from build123d import *

# Parameters (mm, degrees)
SKETCH_1_W                  = 220
SKETCH_1_H                  = 224.25
SKETCH_1_W_2                = 210
SKETCH_1_H_2                = 214.25
EXTRUDE_1_DEPTH             = 310
SKETCH_2_W                  = 280
SKETCH_2_H                  = 284.25
SKETCH_2_W_2                = 210
SKETCH_2_H_2                = 214.25
EXTRUDE_2_DEPTH             = 10
FILLET_1_R                  = 5
FILLET_2_R                  = 5
FILLET_3_R                  = 10
HOLE_WIZARD_8_4_8_4_1_D     = 8.4
MM_11_D                     = 10
HOLE_WIZARD_4_5_4_5_1_D     = 4.5
HOLE_WIZARD_4_5_4_5_1_DEPTH = 5
HOLE_WIZARD_6_6_6_6_1_D     = 6.6
HOLE_WIZARD_6_6_6_6_1_DEPTH = 5
HOLE_WIZARD_5_5_5_5_1_D     = 5.5
HOLE_WIZARD_5_5_5_5_1_DEPTH = 5
CUT_EXTRUDE_1_REACH         = 252
SKETCH_45_W                 = 250
SKETCH_45_H                 = 154.25
FILLET_4_R                  = 5
SKETCH_49_W                 = 256
SKETCH_49_H                 = 160.25
EXTRUDE_3_DEPTH             = 3
FILLET_5_R                  = 5
SKETCH_50_W                 = 216
SKETCH_50_H                 = 220.25
EXTRUDE_4_DEPTH             = 3
FILLET_6_R                  = 5
HOLE_WIZARD_6_4_6_4_1_D     = 6.4
HOLE_WIZARD_6_4_6_4_1_DEPTH = 5
HOLE_WIZARD_4_2_4_2_1_D     = 4.2
HOLE_WIZARD_4_2_4_2_1_DEPTH = 5


with BuildPart() as part:
    # 草图1 → 凸台-拉伸1 (new body)
    with BuildSketch(Plane.XY):
        Rectangle(SKETCH_1_W, SKETCH_1_H)
        Rectangle(SKETCH_1_W_2, SKETCH_1_H_2, mode=Mode.SUBTRACT)
    extrude(amount=EXTRUDE_1_DEPTH)

    # 草图2 → 凸台-拉伸2 (add)
    with BuildSketch(Plane(origin=(0, 0, 0), x_dir=(-1, 0, 0), z_dir=(0, 0, -1))):
        Rectangle(SKETCH_2_W, SKETCH_2_H)
        Rectangle(SKETCH_2_W_2, SKETCH_2_H_2, mode=Mode.SUBTRACT)
    extrude(amount=EXTRUDE_2_DEPTH)

    # 圆角1
    fillet_1_edges = [part.edges().sort_by_distance(p)[0] for p in [
        (110, -112.125, 155),
        (-110, -112.125, 155),
        (-110, 112.125, 155),
        (110, 112.125, 155),
    ]]
    fillet(fillet_1_edges, radius=FILLET_1_R)

    # 圆角2
    fillet_2_edges = [part.edges().sort_by_distance(p)[0] for p in [
        (105, -107.125, 150),
        (105, 107.125, 150),
        (-105, 107.125, 150),
        (-105, -107.125, 150),
    ]]
    fillet(fillet_2_edges, radius=FILLET_2_R)

    # 圆角3
    fillet_3_edges = [part.edges().sort_by_distance(p)[0] for p in [
        (-140, -142.125, -5),
        (-140, 142.125, -5),
        (140, 142.125, -5),
        (140, -142.125, -5),
    ]]
    fillet(fillet_3_edges, radius=FILLET_3_R)

    # Ø8.4 (8.4) 直径孔1 (through all)
    with Locations(Plane.XY):
        with Locations((120, 122.125), (120, -122.125), (-120, -122.125), (-120, 122.125)):
            Hole(HOLE_WIZARD_8_4_8_4_1_D / 2)

    # 大小mm 暗销孔11 (through all)
    with Locations(Plane(origin=(0, 112.125, 0), x_dir=(1, 0, 0), z_dir=(0, 1, 0))):
        with Locations((-75, -165), (-50, -165), (-50, -190), (-75, -190), (50, -190), (50, -165), (75, -165), (75, -190)):
            Hole(MM_11_D / 2)

    # Ø4.5 (4.5) 直径孔1
    with Locations(Plane(origin=(0, 112.125, 0), x_dir=(1, 0, 0), z_dir=(0, 1, 0))):
        with Locations((0, -105), (0, -165), (0, -225), (0, -285)):
            Hole(HOLE_WIZARD_4_5_4_5_1_D / 2, depth=HOLE_WIZARD_4_5_4_5_1_DEPTH)

    # Ø6.6 (6.6) 直径孔1
    with Locations(Plane(origin=(0, -112.125, 0), x_dir=(-1, 0, 0), z_dir=(0, -1, 0))):
        with Locations((19, -105.5), (-19, -105.5)):
            Hole(HOLE_WIZARD_6_6_6_6_1_D / 2, depth=HOLE_WIZARD_6_6_6_6_1_DEPTH)

    # Ø5.5 (5.5) 直径孔1
    with Locations(Plane(origin=(0, -112.125, 0), x_dir=(-1, 0, 0), z_dir=(0, -1, 0))):
        with Locations((15, -280), (-15, -280)):
            Hole(HOLE_WIZARD_5_5_5_5_1_D / 2, depth=HOLE_WIZARD_5_5_5_5_1_DEPTH)

    # 草图45 → 切除-拉伸1 (cut, up to next)
    with BuildSketch(Plane.ZY.offset(110), mode=Mode.PRIVATE) as cut_extrude_1_sk1:
        with Locations((155, 0)):
            Rectangle(SKETCH_45_W, SKETCH_45_H)
    cut_extrude_1_tool1 = extrude(cut_extrude_1_sk1.sketch, amount=-CUT_EXTRUDE_1_REACH, mode=Mode.PRIVATE) & part.part
    add(cut_extrude_1_tool1.solids().sort_by_distance((-110, 0, 155))[0], mode=Mode.SUBTRACT)

    # 圆角4
    fillet_4_edges = [part.edges().sort_by_distance(p)[0] for p in [
        (-107.5, -77.125, 280),
        (-107.5, 77.125, 280),
        (-107.5, 77.125, 30),
        (-107.5, -77.125, 30),
    ]]
    fillet(fillet_4_edges, radius=FILLET_4_R)

    # 草图49 → 凸台-拉伸3 (add)
    with BuildSketch(Plane.ZY.offset(110)):
        with Locations((155, 0)):
            Rectangle(SKETCH_49_W, SKETCH_49_H)
        with BuildLine():
            Line((280, -72.125), (280, 72.125))
            ThreePointArc((280, 72.125), (278.535533906, 75.660533906), (275, 77.125))
            Line((275, 77.125), (35, 77.125))
            ThreePointArc((35, 77.125), (31.464466094, 75.660533906), (30, 72.125))
            Line((30, 72.125), (30, -72.125))
            ThreePointArc((30, -72.125), (31.464466094, -75.660533906), (35, -77.125))
            Line((35, -77.125), (275, -77.125))
            ThreePointArc((275, -77.125), (278.535533906, -75.660533906), (280, -72.125))
        make_face(mode=Mode.SUBTRACT)
    extrude(amount=EXTRUDE_3_DEPTH)

    # 圆角5
    fillet_5_edges = [part.edges().sort_by_distance(p)[0] for p in [
        (-111.5, 80.125, 27),
        (-111.5, -80.125, 27),
        (-111.5, -80.125, 283),
        (-111.5, 80.125, 283),
    ]]
    fillet(fillet_5_edges, radius=FILLET_5_R)

    # 草图50 → 凸台-拉伸4 (add)
    with BuildSketch(Plane(origin=(0, 0, -10), x_dir=(-1, 0, 0), z_dir=(0, 0, -1))):
        Rectangle(SKETCH_50_W, SKETCH_50_H)
        with BuildLine():
            Line((-100, -107.125), (100, -107.125))
            ThreePointArc((100, -107.125), (103.535533906, -105.660533906), (105, -102.125))
            Line((105, -102.125), (105, 102.125))
            ThreePointArc((105, 102.125), (103.535533906, 105.660533906), (100, 107.125))
            Line((100, 107.125), (-100, 107.125))
            ThreePointArc((-100, 107.125), (-103.535533906, 105.660533906), (-105, 102.125))
            Line((-105, 102.125), (-105, -102.125))
            ThreePointArc((-105, -102.125), (-103.535533906, -105.660533906), (-100, -107.125))
        make_face(mode=Mode.SUBTRACT)
    extrude(amount=EXTRUDE_4_DEPTH)

    # 圆角6
    fillet_6_edges = [part.edges().sort_by_distance(p)[0] for p in [
        (108, 110.125, -11.5),
        (108, -110.125, -11.5),
        (-108, -110.125, -11.5),
        (-108, 110.125, -11.5),
    ]]
    fillet(fillet_6_edges, radius=FILLET_6_R)

    # Ø6.4 (6.4) 直径孔1
    with Locations(Plane.ZY.offset(110)):
        with Locations((20, 87.125), (20, -87.125), (290, -87.125), (290, 87.125)):
            Hole(HOLE_WIZARD_6_4_6_4_1_D / 2, depth=HOLE_WIZARD_6_4_6_4_1_DEPTH)

    # Ø4.2 (4.2) 直径孔1
    with Locations(Plane(origin=(0, -107.125, 0), x_dir=(1, 0, 0), z_dir=(0, 1, 0))):
        with Locations((-15, -11.55), (15, -11.55), (15, -41.55), (-15, -41.55)):
            Hole(HOLE_WIZARD_4_2_4_2_1_D / 2, depth=HOLE_WIZARD_4_2_4_2_1_DEPTH)


solid = part.part
Can you work these out from the model? Positions are in its coordinate system, mm. A direction names the side the tool comes from. Coordinates: 2 decimals unless noted, no trailing zeros. Order: outer loops, then holes, each group sorted by start corner. A loop starts at its lowest first (then second) coordinate and runs counter-clockwise, first axis right, second up. Notation, with made-up numbers: (35, -26) -> (82, -26) arc R26 ccw to (82, -8) -> close; hole circle Ø8 at (9, 58.5). An arc over 180 degrees is marked (long way). Use one line per item in the form item = value.
Q1. Imagine slicing it at A-A, the plane x = -50. Give the number of separate pieces and of enclosed holes in the cut face, then the cut area to 3 significant figures.
From the geometry:
separate_pieces = 6
enclosed_holes = 0
area = 3,620 mm²
Q2. We'd pull the mould along Z, two halves only. Please class faces 4 (the face through (55, 110, 165)), 5 (the face through (2, -142.125, -5)): released by +Z, released by -Z, zero draft, split by the parting line, or undercut.
From the geometry:
face_4 = undercut
face_5 = zero draft
Q3. Imagine slicing it at C-C, the plane x = -120. List the corners of the cut face in (y, z) for me (3 decimals).
From the geometry:
outline = (-142.125, -10) -> (-126.325, -10) -> (-126.325, 0) -> (-142.125, 0) -> close; (-117.925, -10) -> (117.925, -10) -> (117.925, 0) -> (-117.925, 0) -> close; (126.325, -10) -> (142.125, -10) -> (142.125, 0) -> (126.325, 0) -> close
Q4. Imagine slicing it at D-D, the plane z = 180. List the corners of the cut face in (x, y) for me (3 decimals), then the cut area to 3 significant figures.
From the geometry:
outline = (-113, -80.125) -> (-110, -80.125) -> (-110, -107.125) arc R5 ccw to (-105, -112.125) -> (105, -112.125) arc R5 ccw to (110, -107.125) -> (110, 107.125) arc R5 ccw to (105, 112.125) -> (-105, 112.125) arc R5 ccw to (-110, 107.125) -> (-110, 80.125) -> (-113, 80.125) -> (-113, 77.125) -> (-105, 77.125) -> (-105, 102.125) arc R5 cw to (-100, 107.125) -> (100, 107.125) arc R5 cw to (105, 102.125) -> (105, -102.125) arc R5 cw to (100, -107.125) -> (-100, -107.125) arc R5 cw to (-105, -102.125) -> (-105, -77.125) -> (-113, -77.125) -> close
area = 3,590 mm²
Q5. I need wall thicknesses on L1, parallel to Z at x = -15, y = -109; L2, parallel to X at y = -111.05, z = 41.55; L3, parallel to Z at x = 50, y = -110. Which ranges of each line are inside material? Lowest first, please.
From the geometry:
L1 = -13 to 9.45, 13.65 to 39.45, 43.65 to 277.25, 282.75 to 310
L2 = -108.1 to -17.1, -12.9 to 12.9, 17.1 to 108.1
L3 = -13 to 160, 170 to 185, 195 to 310
Q6. Imagine slicing it at B-B, the plane y = 20. List the corners of the cut face in (x, z) for me, then the cut area to 3 significant figures.
From the geometry:
outline = (-140, -10) -> (-108, -10) -> (-108, -13) -> (-105, -13) -> (-105, 30) -> (-113, 30) -> (-113, 27) -> (-110, 27) -> (-110, 0) -> (-140, 0) -> close; (-113, 280) -> (-105, 280) -> (-105, 310) -> (-110, 310) -> (-110, 283) -> (-113, 283) -> close; (105, -13) -> (108, -13) -> (108, -10) -> (140, -10) -> (140, 0) -> (110, 0) -> (110, 310) -> (105, 310) -> close
area = 2,590 mm²
Q7. Will these pins go through, and if not, where does the flat tip stop? P1, Ø6.5, axis at x = 120, y = 122.125, coming from the -Z side; P2, Ø1, axis at x = -6.5, z = 259.5, coming from the -Y side (3 decimals); P3, Ø10, axis at y = -108, z = 176, coming from the -X side; P4, Ø9.5, axis at x = 120, y = -122.125, coming from the -Z side.
From the geometry:
P1 = through
P2 = -112.125
P3 = -110
P4 = -10
Q8. Which directions (+Z, -Z, +X, -X, +Y, -Y) give clear straight access to the entire face, cutting with the end or side of a thin tool? Please do faces 1 (the face through (110, -1, 153)), 2 (the face through (2, 142.125, -5)), 3 (the face through (-1, 107.125, 151)).
From the geometry:
face_1 = +Z, +X, +Y, -Y
face_2 = +Z, -Z, +X, -X, +Y
face_3 = +Z, -Z
